Read the model definition and answer for the solid it produces. Units are mm, in the model's axes. A direction names the side the tool comes from. Give positions to 0.01 mm unless a question says otherwise; leave off trailing zeros. Order: outer loops, then holes, each group sorted by start corner. A loop starts at its lowest first (then second) coordinate and runs counter-clockwise, first axis right, second up. Notation, with made-up numbers: M -5,52 L 2,52 A11 cw 2,72 Z; hole C 34,48 d8. An arc over 180 degrees is marked long. One line per item, written item: value.
from build123d import *

# Parameters (mm, degrees)
F0_R     = 59.8445328198
F1_DEPTH = 25.4
F2_R     = 1.6595219512
F2_R_2   = 6.6078081375
F2_R_3   = 9.0128381588
F3_DEPTH = 25.4


with BuildPart() as f1:
    # F0 (on Front) → F1 (new body)
    with BuildSketch(Plane.XZ):
        with Locations((-51.3602979481, 48.6088730395)):
            Circle(F0_R)
    extrude(amount=F1_DEPTH)

    # F2 (on face) → F3 (join)
    with BuildSketch(Plane.XZ.offset(25.4)):
        with BuildLine():
            ThreePointArc((-74.7262415408, 87.5429960215), (-70.6324871698, 83.5455246385), (-69.1296755989, 78.0246406794))
            ThreePointArc((-69.1296755989, 78.0246406794), (-75.594202636, 68.0728078801), (-87.3145593395, 69.9335401611))
            ThreePointArc((-87.3145593395, 69.9335401611), (-85.74951144, 40.3862521604), (-63.8172999639, 20.5249907984))
            ThreePointArc((-63.8172999639, 20.5249907984), (-55.8809359492, 19.0161078752), (-47.8303578802, 18.3446957784))
            ThreePointArc((-47.8303578802, 18.3446957784), (-22.2494316739, 30.6402887159), (-11.8735676311, 57.0582151413))
            ThreePointArc((-11.8735676311, 57.0582151413), (-33.7521367496, 91.9859279311), (-74.7262415408, 87.5429960215))
        make_face()
        with Locations((-76.2917250395, 57.0582151413)):
            Circle(F2_R, mode=Mode.SUBTRACT)
        with Locations((-57.3005713522, 57.0582151413)):
            Circle(F2_R_2, mode=Mode.SUBTRACT)
        with Locations((-33.9007563889, 78.1127512455)):
            Circle(F2_R_3, mode=Mode.SUBTRACT)
        with BuildLine():
            ThreePointArc((-87.3145593395, 69.9335401611), (-88.8832654664, 84.3591256886), (-74.7262415408, 87.5429960215))
            ThreePointArc((-74.7262415408, 87.5429960215), (-33.7521367496, 91.9859279311), (-11.8735676311, 57.0582151413))
            ThreePointArc((-11.8735676311, 57.0582151413), (-22.2494316739, 30.6402887159), (-47.8303578802, 18.3446957784))
            ThreePointArc((-47.8303578802, 18.3446957784), (8.3017992463, 40.0870242253), (31.7662845989, 95.5213622938))
            ThreePointArc((31.7662845989, 95.5213622938), (-93.1100278653, 156.2681263545), (-63.8172999639, 20.5249907984))
            ThreePointArc((-63.8172999639, 20.5249907984), (-85.74951144, 40.3862521604), (-87.3145593395, 69.9335401611))
        make_face()
        with BuildLine():
            ThreePointArc((-47.8303578802, 18.3446957784), (-55.8809359492, 19.0161078752), (-63.8172999639, 20.5249907984))
            ThreePointArc((-63.8172999639, 20.5249907984), (-55.9383572599, 18.5950679887), (-47.8303578802, 18.3446957784))
        make_face()
    extrude(amount=F3_DEPTH)


solid = f1.part
1) Find section A-A, the plane z = 100. Write down the section's boundary in (x, y), plus the area to 3 significant figures.
Reported:
outline: M -122.53,-50.8 L 31.64,-50.8 L 31.64,-25.4 L -20.7,-25.4 L -20.7,0 L -82.02,0 L -82.02,-25.4 L -122.53,-25.4 Z
area: 5,470 mm^2
2) Find section B-B, the plane y = -37. Write down the section's boundary in (x, z) (3 decimals), plus the area to 3 significant figures.
Reported:
outline: M -63.817,20.525 A38.819 ccw -47.83,18.345 A77.213 ccw long Z; hole C -80.022,78.025 d21.785; hole C -76.292,57.058 d3.319; hole C -57.301,57.058 d13.216; hole C -33.901,78.113 d18.026
area: 18,000 mm^2
3) Find section C-C, the plane x = -58.5. Write down the section's boundary in (y, z).
Reported:
outline: M -50.8,19.03 L -25.4,19.03 L -25.4,-10.81 L 0,-10.81 L 0,108.03 L -25.4,108.03 L -25.4,171.62 L -50.8,171.62 L -50.8,63.56 L -25.4,63.56 L -25.4,50.56 L -50.8,50.56 Z
4) Each of these flat-tipped pins is pushed along its axis until it touches: pin 1 Ø6.5 at (x, z) = (-79, 78) entering from -Y; pin 2 Ø4 at (x, y) = (-106.5, -16) entering from -Z; pin 3 Ø6 at (y, z) = (-22.5, 48.5) entering from -X. Where does it stop, or does it pass through?
Reported:
pin 1: stops at y = -25.4
pin 2: stops at z = 21.09
pin 3: stops at x = -111.2
5) Consider probe 1 along Y at (x, z) = (-82, 21.5); probe 2 along Y at (x, z) = (-35, 135); probe 3 along Z at (x, y) = (19, -45.5). Determine where each line is inside the solid, lowest interval first.
Reported:
probe 1: y = -25.4 to 0
probe 2: y = -50.8 to -25.4
probe 3: z = 53 to 138.05
6) Which of the six approach directions +Z, -Z, +X, -X, +Y, -Y give full straight-line access (tool end or side, diameter ignored) to faces 1 (the face through (-56.05, -37.92, 18.61)), 2 (the face through (-34, -25.4, 78)), 3 (the face through (-52, 0, 49)), 4 (the face through (-47, -25.4, 122))?
Reported:
face 1: -Z, -Y
face 2: -Y
face 3: +Z, -Z, +X, -X, +Y
face 4: +Z, +Y
7) Find section D-D, the plane z = 31. Write down the section's boundary in (x, y).
Reported:
outline: M -108.56,-25.4 L -87.86,-25.4 L -87.86,-50.8 L -3.03,-50.8 L -3.03,-25.4 L 5.83,-25.4 L 5.83,0 L -108.56,0 Z
8) Determine the mould class of faces 5 (the face through (-47, -50.8, 97)), 6 (the face through (-64.333, -12.522, -9.813)), 7 (the face through (-54.251, -37.922, 51.196)) for opening direction X: +X half, -X half, draft (parallel to the pull), parting line (faces both ways), or undercut.
Reported:
face 5: draft
face 6: parting line
face 7: undercut
